Geometry check sheet. Reference: the model listing, model coordinates, mm. A direction names the side the tool comes from. Give positions to 0.01 mm unless a question says otherwise; leave off trailing zeros. Order: outer loops, then holes, each group sorted by start corner. A loop starts at its lowest first (then second) coordinate and runs counter-clockwise, first axis right, second up.
from build123d import *

# Parameters (mm, degrees)
SKETCH1_R           = 88.9
SKETCH1_R_2         = 6.35
BOSS_EXTRUDE1_DEPTH = 5.08
SKETCH2_R           = 6.35
BOSS_EXTRUDE2_DEPTH = 11.43
BOSS_EXTRUDE3_START = -50.8
SKETCH3_R           = 6.35
BOSS_EXTRUDE3_DEPTH = 50.8


with BuildPart() as part:
    # Sketch1 → Boss-Extrude1 (new body)
    with BuildSketch(Plane.XY):
        Circle(SKETCH1_R)
        Circle(SKETCH1_R_2, mode=Mode.SUBTRACT)
        with Locations((0, -76.2)):
            Circle(SKETCH1_R_2, mode=Mode.SUBTRACT)
        with Locations((0, 76.2)):
            Circle(SKETCH1_R_2, mode=Mode.SUBTRACT)
    extrude(amount=BOSS_EXTRUDE1_DEPTH)

    # Sketch2 → Boss-Extrude2 (add)
    with BuildSketch(Plane.XY):
        with Locations((0, -76.2)):
            Circle(SKETCH2_R)
    extrude(amount=BOSS_EXTRUDE2_DEPTH)

    # Sketch3 → Boss-Extrude3 (add)
    with BuildSketch(Plane.XY.offset(5.08).offset(BOSS_EXTRUDE3_START)):
        Circle(SKETCH3_R)
    extrude(amount=BOSS_EXTRUDE3_DEPTH)


solid = part.part
Item 1: Gauge pin test, flat ends, axial feed: pin 1 (16.5 mm diameter, centred on x = 0, y = 76.2, fed in from +Z); pin 2 (12 mm diameter, centred on y = -9, z = 2.5, fed in from +X); pin 3 (6 mm diameter, centred on x = 42.5, y = -52.5, fed in from -Z). Record the tip position at first contact, or that the pin passes through.
Reported:
pin 1: stops at z = 5.08
pin 2: stops at x = 88.85
pin 3: stops at z = 0
Item 2: Draft check along X on faces 1 (the cylindrical face through (-1.38, 70, 2.5)), 2 (the cylindrical face through (84.795, 26.703, 2.504)), 3 (the flat face through (0, 0, -45.72)). Enter one of: released by +X, released by -X, zero draft, split by the parting line, or undercut.
Reported:
face 1: undercut
face 2: split by the parting line
face 3: zero draft
Item 3: Scan lines: L1, parallel to Y at x = 0, z = 2; L2, parallel to Z at x = -4, y = 60.5; L3, parallel to Y at x = 66, z = 2. Record each from-to range of solid material in increasing order.
Reported:
L1: y = -88.9 to 69.85, 82.55 to 88.9
L2: z = 0 to 5.08
L3: y = -59.56 to 59.56
Item 4: Sectioned sample at D-D (z = -9). Enter the section's corners in (x, y).
Reported:
outline: circle Ø12.7 at (0, 0)
Item 5: Sectioned sample at A-A (x = 0). Enter the section's corners in (y, z), and give its area (3 significant figures).
Reported:
outline: (-88.9, 0) - (-6.35, 0) - (-6.35, -45.72) - (6.35, -45.72) - (6.35, 0) - (69.85, 0) - (69.85, 5.08) - (-69.85, 5.08) - (-69.85, 11.43) - (-82.55, 11.43) - (-82.55, 5.08) - (-88.9, 5.08) - close; (82.55, 0) - (88.9, 0) - (88.9, 5.08) - (82.55, 5.08) - close
area: 1,500 mm2
Item 6: Set-up check for faces 4 (the cylindrical face through (-1.38, -6.2, -23.18)), 5 (the cylindrical face through (3.414, -70.846, 8.211)), 6 (the flat face through (0, -76, 11.43)): record each of +Z, -Z, +X, -X, +Y, -Y from which the full face is reachable in a straight line by a thin tool's end or side.
Reported:
face 4: -Z
face 5: +Z
face 6: +Z, +X, -X, +Y, -Y
Item 7: Sectioned sample at B-B (y = 76.2). Enter the section's corners in (x, z).
Reported:
outline: (-45.79, 0) - (-6.35, 0) - (-6.35, 5.08) - (-45.79, 5.08) - close; (6.35, 0) - (45.79, 0) - (45.79, 5.08) - (6.35, 5.08) - close
Item 8: Sectioned sample at C-C (y = 0). Enter the section's corners in (x, z).
Reported:
outline: (-88.9, 0) - (-6.35, 0) - (-6.35, -45.72) - (6.35, -45.72) - (6.35, 0) - (88.9, 0) - (88.9, 5.08) - (-88.9, 5.08) - close
